```python
from build123d import *

# Parameters (mm, degrees)
SKETCH_2_R      = 1
EXTRUDE_1_DEPTH = 27


with BuildPart() as part:
    # 草图1 → 旋转1 (revolve)
    with BuildSketch(Plane.XY, mode=Mode.PRIVATE) as revolve_1_sk:
        Polygon((20, 0), (28, 0), (28, 3.662344451), (33, 3.662344451), (33, 0), (41, 0), (41, 12), (33, 12), (33, 8.337655549), (28, 8.337655549), (28, 11.96151904), (20, 11.96151904), align=None)
    revolve(revolve_1_sk.sketch.rotate(Axis((0, 0, 0), (0, 1, 0)), 90), axis=Axis((0, 0, 0), (0, 1, 0)))

    # 草图2 → 凸台-拉伸1 (add)
    with BuildSketch(Plane.XZ):
        with Locations(Location((0.996647287, 39.458172136, 0), (0, 0, 270))):
            Circle(SKETCH_2_R)
    extrude(amount=EXTRUDE_1_DEPTH)


solid = part.part
```
Input: part model. Units: mm. Frame: model coordinates. A direction names the side the tool comes from. Coordinates: 2 decimals unless noted, no trailing zeros. Loops run counter-clockwise (first coordinate to the right, second up) from the corner with the lowest first, then second, coordinate; pieces in that order, holes last. Notation, with made-up numbers: (8.25, 8) - (21.25, 8) arc R12 cw to (21.25, 22) - close; hole circle Ø11 at (55.25, 87). An arc over 180 degrees is marked (long way). Answer in a Markdown table with one row per item.
(1) Cut plane D-D on z = -23.5. Output: boundary loops of the cut face in (x, y), plus the area to 3 significant figures.
Model answer:
| item | result |
|---|---|
| outline | (-33.6, 0) - (-23.17, 0) - (-23.17, 3.66) - (-15.22, 3.66) - (-15.22, 0) - (15.22, 0) - (15.22, 3.66) - (23.17, 3.66) - (23.17, 0) - (33.6, 0) - (33.6, 12) - (23.17, 12) - (23.17, 8.34) - (15.22, 8.34) - (15.22, 11.96) - (-15.22, 11.96) - (-15.22, 8.34) - (-23.17, 8.34) - (-23.17, 12) - (-33.6, 12) - close |
| area | 689 mm² |
(2) Material intervals for L1, parallel to X at y = 10, z = 0; L2, parallel to X at y = 1.5, z = -22; L3, parallel to X at y = 3.75, z = 0, sorted ascending. Write a range as from..to.
Model answer:
| item | result |
|---|---|
| L1 | x = -41..-33, -28..-20, 20..28, 33..41 |
| L2 | x = -34.6..-24.6, -17.32..17.32, 24.6..34.6 |
| L3 | x = -41..-20, 20..41 |
(3) Cut plane A-A on z = 0. Output: boundary loops of the cut face in (x, y), plus the area to 3 significant figures.
Model answer:
| item | result |
|---|---|
| outline | (-41, 0) - (-33, 0) - (-33, 3.66) - (-28, 3.66) - (-28, 0) - (-20, 0) - (-20, 11.96) - (-28, 11.96) - (-28, 8.34) - (-33, 8.34) - (-33, 12) - (-41, 12) - close; (20, 0) - (28, 0) - (28, 3.66) - (33, 3.66) - (33, 0) - (41, 0) - (41, 12) - (33, 12) - (33, 8.34) - (28, 8.34) - (28, 11.96) - (20, 11.96) - close |
| area | 430 mm² |
(4) Cut plane C-C on y = 9.5. Output: boundary loops of the cut face in (x, z).
Model answer:
| item | result |
|---|---|
| outline | circle Ø82 at (0, 0); circle Ø56 at (0, 0); hole circle Ø66 at (0, 0); hole circle Ø40 at (0, 0) |
(5) Cut plane B-B on x = -8.5. Output: boundary loops of the cut face in (y, z).
Model answer:
| item | result |
|---|---|
| outline | (0, -40.11) - (12, -40.11) - (12, -31.89) - (8.34, -31.89) - (8.34, -26.68) - (11.96, -26.68) - (11.96, -18.1) - (0, -18.1) - (0, -26.68) - (3.66, -26.68) - (3.66, -31.89) - (0, -31.89) - close; (0, 18.1) - (11.96, 18.1) - (11.96, 26.68) - (8.34, 26.68) - (8.34, 31.89) - (12, 31.89) - (12, 40.11) - (0, 40.11) - (0, 31.89) - (3.66, 31.89) - (3.66, 26.68) - (0, 26.68) - close |
(6) Pin query (flat end, axial travel): P1, Ø12, axis at y = -1, z = -22, coming from the +X side; P2, Ø24.5, axis at x = -3, z = 11, coming from the -Y side; P3, Ø10, axis at x = 17.5, z = -9.5, coming from the +Y side. Return the tip coordinate at first contact, or that it passes through.
Model answer:
| item | result |
|---|---|
| P1 | stops at x = 37.71 |
| P2 | stops at y = 0 |
| P3 | stops at y = 11.96 |
(7) Mould query, pull axis Z, two halves, no side actions, for faces 4 (the face through (-18, 0, -28)), 5 (the face through (-9.912, 10.143, -31.476)), 6 (the face through (1.297, -13.311, 38.504)). Classes: pulls with the +Z half, pulls with the -Z half, needs draft (parallel to the pull), parting line crosses it, or undercut.
Model answer:
| item | result |
|---|---|
| face 4 | needs draft |
| face 5 | undercut |
| face 6 | parting line crosses it |
(8) Set-up query: faces 1 (the face through (24.84, 1.86, -12.92)), 2 (the face through (-0.88, 5.9, 19.98)), 3 (the face through (24, 8.338, 15)). Return all of +Z, -Z, +X, -X, +Y, -Y with unobstructed straight access to the full face (end or side cutting, diameter ignored); none if empty.
Model answer:
| item | result |
|---|---|
| face 1 | -Y |
| face 2 | +Y, -Y |
| face 3 | +Y |
